Autodesk Inventor part; units mm, degrees
ref_plane "YZ Plane" through (0, 0, 0) normal (1, 0, 0) x (0, 1, 0)
ref_plane "XZ Plane" through (0, 0, 0) normal (0, 1, 0) x (-1, 0, 0)
ref_plane "XY Plane" through (0, 0, 0) normal (0, 0, 1) x (1, 0, 0)
sketch "Skizze1" plane through (0, 0, 0) normal (0, 0, 1) x (1, 0, 0)
  line L0 (-7, 0) -> (7, 0)
  line L1 (0, -7) -> (0, 7)
  circle A0 centre (0, 0) radius 5
  dimension "d0" = 10
extrude "Extrusion1" add sketch "Skizze1" along normal blind 44
sketch "Skizze2" plane through (0, 0, 44) normal (0, 0, 1) x (1, 0, 0)
  circle A0 centre (0, 0) radius 5
  circle A1 centre (0, 0) radius 4.25
  dimension "d3" = 8.5
extrude "Extrusion2" add sketch "Skizze2" along normal blind 11 contours A1
sketch "Skizze3" plane through (0, 0, 0) normal (0, 0, -1) x (-1, 0, 0)
  circle A0 centre (0, 0) radius 5
hole "Bohrung1" at (0, 0, 0) direction (0, 0, 1) diameter 4.134 depth 14.2 tip angle 118
sketch "Skizze4" plane through (0, 0, 55) normal (0, 0, 1) x (1, 0, 0)
  line L0 (3, -3) -> (-3, -3)
  line L1 (-3, -3) -> (-3, 3)
  line L2 (-3, 3) -> (3, 3)
  line L3 (3, 3) -> (3, -3)
  circle A0 centre (0, 0) radius 4.25
  line L4 (3, -3) -> (-3, 3) construction
  line L5 (-3, -3) -> (3, 3) construction
  dimension "d13" = 6
  dimension "d14" = 6
extrude "Extrusion3" add sketch "Skizze4" along normal blind 5 contours L0 L1 L2 L3
sketch "Skizze5" plane through (0, 0, 0) normal (0, 1, 0) x (-1, 0, 0)
  line L0 (0, -12.3) -> (0, 73.8)
  line L1 (7, 0) -> (-7, 0)
  line L2 (8.228, 20) -> (-9.772, 20)
  line L3 (5, 44) -> (-5, 44)
  line L4 (5, 0) -> (-5, 0)
  line L5 (5, 0) -> (5, 44)
  line L6 (-5, 0) -> (-5, 44)
  line L7 (4, 16) -> (5, 16)
  line L8 (5, 16) -> (5, 24)
  line L9 (5, 24) -> (4, 24)
  line L10 (4, 24) -> (4, 16)
  line L11 (4, 16) -> (5, 24) construction
  line L12 (5, 16) -> (4, 24) construction
  line L13 (-4, 16) -> (-5, 16)
  line L14 (-5, 16) -> (-5, 24)
  line L15 (-5, 24) -> (-4, 24)
  line L16 (-4, 24) -> (-4, 16)
  line L17 (-4, 16) -> (-5, 24) construction
  line L18 (-5, 16) -> (-4, 24) construction
  point P0 (0, 0)
  point P1 (4.5, 20)
  point P2 (-4.5, 20)
  dimension "d17" = 8
  dimension "d18" = 8
  dimension "d19" = 20
extrude "Extrusion4" cut sketch "Skizze5" along normal mid plane 44 contours L10 L9 L5 L2 | L2 L5 L7 L10 | L16 L13 L6 L2 | L2 L6 L15 L16
equation "\"d13\" = d14"
properties part number "24_0497_009"
Build history of the part. All positions in model axes, mm. A direction names the side the tool comes from. Round coordinates to 2 decimals unless told otherwise and drop trailing zeros. Order: outer loops, then holes, each group sorted by start corner. A loop starts at its lowest first (then second) coordinate and runs counter-clockwise, first axis right, second up. Notation, with made-up numbers: (59, -35.75) - (101, -35.75) arc R16 cw to (101, -19.75) - close; hole circle Ø8 at (44, -15). An arc over 180 degrees is marked (long way). Use a Markdown table: item, result.
1) Wall check: L1, parallel to X at y = 0, z = 7.5; L2, parallel to Z at x = -1.25, y = -3.25. Give the ranges that are in metal, low to high.
Recorded:
| item | result |
|---|---|
| L1 | x = -5 to -2.07, 2.07 to 5 |
| L2 | z = 0 to 55 |
2) Pull direction Z, two halves, no side cores. Call faces 1 (the face through (2, -1, 0)), 2 (the face through (-4, 0, 20)), 3 (the face through (1.26, -1.64, 7.2)): pulls with the +Z half, pulls with the -Z half, needs draft (parallel to the pull), parting line crosses it, or undercut.
Recorded:
| item | result |
|---|---|
| face 1 | pulls with the -Z half |
| face 2 | undercut |
| face 3 | needs draft |
3) Saw through at B-B on x = 3.5. Write the cut outline in (y, z).
Recorded:
| item | result |
|---|---|
| outline | (-3.57, 0) - (3.57, 0) - (3.57, 44) - (2.41, 44) - (2.41, 55) - (-2.41, 55) - (-2.41, 44) - (-3.57, 44) - close |
4) Flat gauge pins, fed straight in: pin 1 Ø3 at (y, z) = (2.5, 11) entering from +X; pin 2 Ø5 at (x, z) = (-0.5, 43) entering from +Y; pin 3 Ø4 at (x, z) = (1.5, 57.5) entering from -Y; pin 4 Ø5 at (y, z) = (-1.5, 21) entering from +X. Where does each tip first touch, or does it go through?
Recorded:
| item | result |
|---|---|
| pin 1 | stops at x = 4.9 |
| pin 2 | stops at y = 5 |
| pin 3 | stops at y = -3 |
| pin 4 | stops at x = 4 |
5) Tool access for faces 4 (the face through (2.285, -3.584, 49.423)), 5 (the face through (0, -3, 57)), 6 (the face through (0, 3, 57)): list every direction of +Z, -Z, +X, -X, +Y, -Y with a clear straight run to the whole face (end or side of a thin tool).
Recorded:
| item | result |
|---|---|
| face 4 | +Z |
| face 5 | +Z, +X, -X, -Y |
| face 6 | +Z, +X, -X, +Y |
6) Saw through at A-A on y = 3.75. Write the cut outline in (x, z), and give its area (3 significant figures).
Recorded:
| item | result |
|---|---|
| outline | (-3.31, 0) - (3.31, 0) - (3.31, 44) - (2, 44) - (2, 55) - (-2, 55) - (-2, 44) - (-3.31, 44) - close |
| area | 335 mm² |
7) Saw through at C-C on z = 31.5. Write the cut outline in (x, y), and give its area (3 significant figures).
Recorded:
| item | result |
|---|---|
| outline | circle Ø10 at (0, 0) |
| area | 78.5 mm² |
